Check sheet for the modelled part. Datum: model origin and axes. Units: mm. A direction names the side the tool comes from. Round coordinates to 2 decimals unless told otherwise and drop trailing zeros. Loops run counter-clockwise (first coordinate to the right, second up) from the corner with the lowest first, then second, coordinate; pieces in that order, holes last. Notation, with made-up numbers: (24, 27.5) - (71, 27.5) arc R16 cw to (71, 50.5) - close; hole circle Ø2 at (15, 33.25). An arc over 180 degrees is marked (long way). Answer in a Markdown table with one row per item. Add a question column.
(1) Access from +Z, -Z, +X, -X, +Y, -Y to the whole of each face (thin tool, end or side, straight path). Record for faces 4 (the flat face through (-6.6, -19.3, -12.2)), 5 (the flat face through (11.455, -301, 0)).
(2) Cross-section at B-B on x = 5.25. Enter the section's corners in (y, z), then the cut area to 3 significant figures.
(3) Thickness scan on line 1 along Z through (x, y) = (-2.5, -493). Record the ranges inside material, lowest first.
(4) Mould release check, pull along X, two halves, no side actions. Record for faces 1 (the flat face through (0, -301, 12.7)), 2 (the flat face through (-11.455, -301, 0)), 3 (the flat face through (12.7, -301, 0)): +X half, -X half, draft (parallel to the pull), parting line (faces both ways), or undercut.
(5) Cross-section at A-A on z = 0. Enter the section's corners in (x, y), then the cut area to 3 significant figures.
(6) Cross-section at C-C on y = -519. Enter the section's corners in (x, z), then the cut area to 3 significant figures.
(7) Gauge pin test, flat end, axial feed: pin 1 (4 mm diameter, centred on x = -8, z = -5, fed in from +Y). Record the tip position at first contact, or that the pin passes through.
from build123d import *

# Parameters (mm, degrees)
F0_W     = 25.4
F0_H     = 25.4
F0_W_2   = 22.9108
F0_H_2   = 22.9108
F1_DEPTH = 609.6
F3_DEPTH = 25.401
F5_DEPTH = 25.401


with BuildPart() as f1:
    # F0 (on Front) → F1 (new body)
    with BuildSketch(Plane.XZ):
        Rectangle(F0_W, F0_H)
        Rectangle(F0_W_2, F0_H_2, mode=Mode.SUBTRACT)
    extrude(amount=F1_DEPTH)

    # F2 (on face) → F3 (cut, through all)
    with BuildSketch(Plane.XY.offset(12.7)):
        Polygon((-12.7, -25.4), (12.7, 0), (-12.7, 0), align=None)
        Polygon((-12.7, -609.6), (12.7, -609.6), (-12.7, -584.2), align=None)
    extrude(amount=-F3_DEPTH, mode=Mode.SUBTRACT)

    # F4 (on face) → F5 (cut, through all)
    with BuildSketch(Plane.YZ.offset(12.7)):
        Polygon((-609.6, 12.7), (-609.6, -12.7), (-584.2, 12.7), align=None)
        Polygon((-25.4, 12.7), (0, -12.7), (0, 12.7), align=None)
    extrude(amount=-F5_DEPTH, mode=Mode.SUBTRACT)


solid = f1.part
Answers:
| question | item | result |
|---|---|---|
| 1 | face 4 | +Z, -Z, -X, +Y |
| 1 | face 5 | +Y, -Y |
| 2 | outline | (-602.15, -12.7) - (-7.45, -12.7) - (-7.45, -11.46) - (-602.15, -11.46) - close; (-585.44, 11.46) - (-24.16, 11.46) - (-25.4, 12.7) - (-584.2, 12.7) - close |
| 2 | area | 1,440 mm^2 |
| 3 | line 1 | z = -12.7 to -11.46, 11.46 to 12.7 |
| 4 | face 1 | draft |
| 4 | face 2 | undercut |
| 4 | face 3 | +X half |
| 5 | outline | (-12.7, -584.2) - (-11.46, -585.44) - (-11.46, -24.16) - (-12.7, -25.4) - close; (11.46, -596.9) - (12.7, -596.9) - (12.7, -12.7) - (11.46, -12.7) - close |
| 5 | area | 1,420 mm^2 |
| 6 | outline | (-12.7, -12.7) - (12.7, -12.7) - (12.7, 12.7) - (-12.7, 12.7) - close; hole (-11.46, -11.46) - (11.46, -11.46) - (11.46, 11.46) - (-11.46, 11.46) - close |
| 6 | area | 120 mm^2 |
| 7 | pin 1 | passes through |
